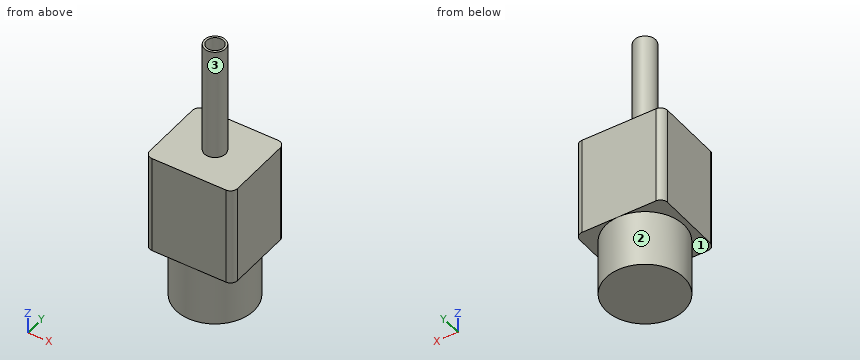
Autodesk Fusion 360 part; units mm, degrees
sketch "Sketch1" plane through (0, 0, 0) normal (0, 0, 1) x (1, 0, 0)
  circle A0 centre (0, 0) radius 27.5
  dimension "d1" = 55
extrude "Extrude1" add sketch "Sketch1" along normal blind 40
sketch "Sketch2" plane through (0, 0, 40) normal (0, 0, 1) x (-1, 0, 0)
  circle A0 centre (0, 0) radius 27.5
  line L0 (0, -27.5) -> (-31, -27.5)
  line L1 (-31, -27.5) -> (-31, 40.6198)
  line L2 (0, 27.5) -> (-33.618, 27.5)
  line L3 (0, -27.5) -> (31, -27.5)
  line L4 (31, -27.5) -> (31, 43)
  line L5 (0, 27.5) -> (37, 27.5)
  dimension "d4" = 90
  dimension "d5" = 31
extrude "Extrude2" add sketch "Sketch2" along normal blind 70
sketch "Sketch3" plane through (0, 0, 110) normal (0, 0, 1) x (-1, 0, 0)
  line L0 (-31, -27.5) -> (31, -27.5)
  line L1 (31, -27.5) -> (31, 27.5)
  line L2 (31, 27.5) -> (-31, 27.5)
  line L3 (-31, 27.5) -> (-31, -27.5)
  circle A0 centre (0, 0) radius 7.5
  dimension "d8" = 15
extrude "Extrude3" add sketch "Sketch3" along normal blind 80 contours A0
sketch "Sketch4" plane through (0, 0, 0) normal (0, 1, 0) x (1, 0, 0)
sketch "Sketch5" plane through (0, 0, 190) normal (0, 0, 1) x (-1, 0, 0)
  circle A0 centre (0, 0) radius 7.5
  circle A1 centre (0, 0) radius 6
  dimension "d14" = 12
extrude "Extrude4" cut sketch "Sketch5" against normal blind 15 contours A1
fillet "Fillet2" radius 5 4 edges at (-31, -27.5, 75) (31, -27.5, 75) (31, 27.5, 75) (-31, 27.5, 75)
Input: part model. Units: mm. Frame: model coordinates. Face numbers are marked on the shaded views. A direction names the side the tool comes from. Coordinates: 2 decimals unless noted, no trailing zeros. Loops run counter-clockwise (first coordinate to the right, second up) from the corner with the lowest first, then second, coordinate; pieces in that order, holes last. Notation, with made-up numbers: M -21.75,-8 L 12.25,-8 A13 cw 12.25,5 Z; hole C -14.5,59 d7. An arc over 180 degrees is marked long. Use a Markdown table: item, result. Add a question column.
1) Section C-C, the plane z = 34.5. Return the cut outline in (x, y).
2) Pin query (flat end, axial travel): P1, Ø8, axis at x = -17.5, z = 116.5, coming from the +Y side; P2, Ø6, axis at x = -2.5, y = 1.5, coming from the +Z side; P3, Ø12, axis at x = -21, y = 10, coming from the +Z side; P4, Ø5, axis at y = -5, z = 36.5, coming from the -X side. Return the tip coordinate at first contact, or that it passes through.
3) Section B-B, the plane x = 19. Return the cut outline in (y, z), plus the area to 3 significant figures.
4) Set-up query: the marked faces 1, 2 and 3. Return all of +Z, -Z, +X, -X, +Y, -Y with unobstructed straight access to the full face (end or side cutting, diameter ignored); none if empty.
5) Section A-A, the plane y = 0. Return the cut outline in (x, z), plus the area to 3 significant figures.
6) Section D-D, the plane x = -20. Return the cut outline in (y, z).
7) Line query: L1, parallel to X at y = 0, z = 180; L2, parallel to Z at x = -10.5, y = -5. Output: solid intervals per line, ascending. Write a range as from..to.
Answer below:
| question | item | result |
|---|---|---|
| 1 | outline | C 0,0 d55 |
| 2 | P1 | through |
| 2 | P2 | z = 175 |
| 2 | P3 | z = 110 |
| 2 | P4 | x = -27.39 |
| 3 | outline | M -27.5,40 L -19.88,40 L -19.88,0 L 19.88,0 L 19.88,40 L 27.5,40 L 27.5,110 L -27.5,110 Z |
| 3 | area | 5,440 mm2 |
| 4 | face 1 | -Z, -X |
| 4 | face 2 | -Z |
| 4 | face 3 | +Z |
| 5 | outline | M -31,40 L -27.5,40 L -27.5,0 L 27.5,0 L 27.5,40 L 31,40 L 31,110 L 7.5,110 L 7.5,190 L 6,190 L 6,175 L -6,175 L -6,190 L -7.5,190 L -7.5,110 L -31,110 Z |
| 5 | area | 7,560 mm2 |
| 6 | outline | M -27.5,40 L -18.87,40 L -18.87,0 L 18.87,0 L 18.87,40 L 27.5,40 L 27.5,110 L -27.5,110 Z |
| 7 | L1 | -7.5..-6, 6..7.5 |
| 7 | L2 | 0..110 |
